The model under review builds one solid part; all positions refer to its coordinate system, in mm. Face numbers are marked on the shaded views. A direction names the side the tool comes from. Coordinates: 2 decimals unless noted, no trailing zeros. Loops run counter-clockwise (first coordinate to the right, second up) from the corner with the lowest first, then second, coordinate; pieces in that order, holes last. Notation, with made-up numbers: (14.25, 24.5) - (49.25, 24.5) arc R14 ccw to (49.25, 30.5) - close; hole circle Ø6 at (54, -11). An arc over 180 degrees is marked (long way). Answer in a Markdown table with one row per item. Add a question column.
(1) For line 1 along X through (y, z) = (55, 6); line 2 along X through (y, z) = (40, 4.25); line 3 along Y through (x, z) = (21, 1.35), list the stretches that pass through material, from the lowest coordinate up.
(2) We need section D-D on x = 21. Write out the cut boundary in (y, z).
(3) We need section A-A on z = 1.5. Give the number of separate pieces and of enclosed holes in the cut face, plus the area to 3 significant figures.
(4) We need section C-C on y = 30. Write out the cut boundary in (x, z).
(5) We need section B-B on x = 41. Write out the cut boundary in (y, z).
(6) Machinability: for the marked faces 4, 5 and 6, which of the approach directions +Z, -Z, +X, -X, +Y, -Y give a long, thin tool a straight path to every point of the face, cutting with its end or side? Answer none if there is none.
(7) For P1, Ø1.9, axis at x = 70, y = 20.5, coming from the -Z side; P2, Ø5.5, axis at x = 21, y = 69, coming from the +Z side; P3, Ø1.5, axis at x = 9, z = 4, coming from the +Y side; P4, Ø2.5, axis at x = 21, y = 9, coming from the -Z side, all flat-tipped, find the tip position at first contact; note any pin that passes through.
(8) Mouldability with a two-part tool opening along X and no side actions: class the marked faces 1, 2 and 3 as +X half, -X half, draft (parallel to the pull), parting line (faces both ways), or undercut.
from build123d import *

# Parameters (mm, degrees)
F1_DEPTH  = 8.5
F2_W      = 70
F2_H      = 68
F2_R      = 30
F3_DEPTH  = 4
F5_DEPTH  = 25
F6_R      = 3.2
F6_R_2    = 1.7
F7_DEPTH  = 3.1
F8_R      = 1.65
F9_DEPTH  = 25
F10_R     = 3.15
F11_DEPTH = 3.1
F13_DEPTH = 25


with BuildPart() as f1:
    # F0 (on Top) → F1 (new body)
    with BuildSketch(Plane.XY):
        with BuildLine():
            Line((0, 78), (0, 39))
            Line((0, 39), (11, 39))
            ThreePointArc((11, 39), (41, 69), (71, 39))
            Line((71, 39), (82, 39))
            Line((82, 39), (82, 78))
            Line((82, 78), (81, 78))
            ThreePointArc((81, 78), (79.535534, 74.464466), (76, 73))
            Line((76, 73), (6, 73))
            ThreePointArc((6, 73), (2.464466, 74.464466), (1, 78))
            Line((1, 78), (0, 78))
        make_face()
        with BuildLine():
            Line((0, 39), (0, 0))
            Line((0, 0), (1, 0))
            ThreePointArc((1, 0), (2.464466, 3.535534), (6, 5))
            Line((6, 5), (76, 5))
            ThreePointArc((76, 5), (79.535534, 3.535534), (81, 0))
            Line((81, 0), (82, 0))
            Line((82, 0), (82, 39))
            Line((82, 39), (71, 39))
            ThreePointArc((71, 39), (41, 9), (11, 39))
            Line((11, 39), (0, 39))
        make_face()
    extrude(amount=F1_DEPTH)

    # F2 (on face) → F3 (cut)
    with BuildSketch(Plane.XY.offset(8.5)):
        with Locations((41, 39)):
            Rectangle(F2_W, F2_H)
        with Locations((41, 39)):
            Circle(F2_R, mode=Mode.SUBTRACT)
    extrude(amount=-F3_DEPTH, mode=Mode.SUBTRACT)

    # F4 (on face) → F5 (cut)
    with BuildSketch(Plane(origin=(0, 0, 0), x_dir=(1, 0, 0), z_dir=(0, 0, -1))):
        with BuildLine():
            ThreePointArc((14.2, -19), (11.297918, -17.797918), (12.5, -20.7))
            ThreePointArc((12.5, -20.7), (13.702082, -20.202082), (14.2, -19))
        make_face()
        with BuildLine():
            ThreePointArc((14.2, -59), (13.702082, -57.797918), (12.5, -57.3))
            ThreePointArc((12.5, -57.3), (11.297918, -60.202082), (14.2, -59))
        make_face()
        with BuildLine():
            ThreePointArc((71.2, -59), (70.702082, -57.797918), (69.5, -57.3))
            ThreePointArc((69.5, -57.3), (68.297918, -60.202082), (71.2, -59))
        make_face()
        with BuildLine():
            ThreePointArc((71.2, -19), (69.5, -17.3), (67.8, -19))
            ThreePointArc((67.8, -19), (68.297918, -20.202082), (69.5, -20.7))
            ThreePointArc((69.5, -20.7), (70.702082, -20.202082), (71.2, -19))
        make_face()
    extrude(amount=-F5_DEPTH, mode=Mode.SUBTRACT)

    # F6 (on face) → F7 (cut)
    with BuildSketch(Plane(origin=(0, 0, 0), x_dir=(1, 0, 0), z_dir=(0, 0, -1))):
        with Locations((12.5, -19)):
            Circle(F6_R)
        with Locations((12.5, -19)):
            Circle(F6_R_2, mode=Mode.SUBTRACT)
        with Locations((12.5, -59)):
            Circle(F6_R)
        with Locations((12.5, -59)):
            Circle(F6_R_2, mode=Mode.SUBTRACT)
        with Locations((69.5, -19)):
            Circle(F6_R)
        with Locations((69.5, -19)):
            Circle(F6_R_2, mode=Mode.SUBTRACT)
        with Locations((69.5, -59)):
            Circle(F6_R)
        with Locations((69.5, -59)):
            Circle(F6_R_2, mode=Mode.SUBTRACT)
    extrude(amount=-F7_DEPTH, mode=Mode.SUBTRACT)

    # F8 (on face) → F9 (cut)
    with BuildSketch(Plane(origin=(0, 0, 0), x_dir=(1, 0, 0), z_dir=(0, 0, -1))):
        with Locations((21, -69)):
            Circle(F8_R)
        with BuildLine():
            ThreePointArc((62.65, -69), (62.166726, -67.833274), (61, -67.35))
            Line((61, -67.35), (61, -69))
            Line((61, -69), (59.35, -69))
            ThreePointArc((59.35, -69), (61, -70.65), (62.65, -69))
        make_face()
        with BuildLine():
            Line((61, -69), (61, -67.35))
            ThreePointArc((61, -67.35), (59.833274, -67.833274), (59.35, -69))
            Line((59.35, -69), (61, -69))
        make_face()
        with BuildLine():
            ThreePointArc((62.65, -9), (61, -7.35), (59.35, -9))
            Line((59.35, -9), (61, -9))
            Line((61, -9), (61, -10.65))
            ThreePointArc((61, -10.65), (62.166726, -10.166726), (62.65, -9))
        make_face()
        with BuildLine():
            Line((61, -9), (59.35, -9))
            ThreePointArc((59.35, -9), (59.833274, -10.166726), (61, -10.65))
            Line((61, -10.65), (61, -9))
        make_face()
        with Locations((21, -9)):
            Circle(F8_R)
    extrude(amount=-F9_DEPTH, mode=Mode.SUBTRACT)

    # F10 (on face) → F11 (cut)
    with BuildSketch(Plane(origin=(0, 0, 0), x_dir=(1, 0, 0), z_dir=(0, 0, -1))):
        with Locations((21, -9)):
            Circle(F10_R)
        with Locations((61, -9)):
            Circle(F10_R)
        with Locations((61, -69)):
            Circle(F10_R)
        with Locations((21, -69)):
            Circle(F10_R)
    extrude(amount=-F11_DEPTH, mode=Mode.SUBTRACT)

    # F12 (on face) → F13 (cut)
    with BuildSketch(Plane(origin=(0, 0, 0), x_dir=(1, 0, 0), z_dir=(0, 0, -1))):
        with BuildLine():
            ThreePointArc((12.5, -9), (9.93934, -7.93934), (11, -10.5))
            Line((11, -10.5), (11, -9))
            Line((11, -9), (12.5, -9))
        make_face()
        with BuildLine():
            Line((11, -9), (11, -10.5))
            ThreePointArc((11, -10.5), (12.06066, -10.06066), (12.5, -9))
            Line((12.5, -9), (11, -9))
        make_face()
        with BuildLine():
            ThreePointArc((69.5, -9), (69.93934, -10.06066), (71, -10.5))
            Line((71, -10.5), (71, -9))
            Line((71, -9), (69.5, -9))
        make_face()
        with BuildLine():
            Line((71, -9), (71, -10.5))
            ThreePointArc((71, -10.5), (72.06066, -10.06066), (72.5, -9))
            ThreePointArc((72.5, -9), (71, -7.5), (69.5, -9))
            Line((69.5, -9), (71, -9))
        make_face()
        with BuildLine():
            ThreePointArc((71, -67.5), (69.93934, -67.93934), (69.5, -69))
            Line((69.5, -69), (71, -69))
            Line((71, -69), (71, -67.5))
        make_face()
        with BuildLine():
            Line((71, -69), (69.5, -69))
            ThreePointArc((69.5, -69), (71, -70.5), (72.5, -69))
            ThreePointArc((72.5, -69), (72.06066, -67.93934), (71, -67.5))
            Line((71, -67.5), (71, -69))
        make_face()
        with BuildLine():
            ThreePointArc((11, -67.5), (9.93934, -70.06066), (12.5, -69))
            Line((12.5, -69), (11, -69))
            Line((11, -69), (11, -67.5))
        make_face()
        with BuildLine():
            Line((11, -69), (12.5, -69))
            ThreePointArc((12.5, -69), (12.06066, -67.93934), (11, -67.5))
            Line((11, -67.5), (11, -69))
        make_face()
    extrude(amount=-F13_DEPTH, mode=Mode.SUBTRACT)


solid = f1.part
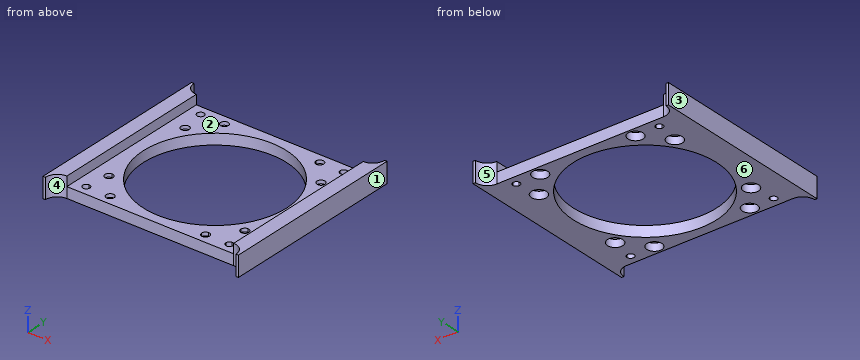
Outcome:
| question | item | result |
|---|---|---|
| 1 | line 1 | 0 to 6, 76 to 82 |
| 1 | line 2 | 0 to 11.02, 70.98 to 82 |
| 1 | line 3 | 5 to 5.85, 12.15 to 16.64, 61.36 to 65.85, 72.15 to 73 |
| 2 | outline | (5, 0) - (5.85, 0) - (5.85, 3.1) - (7.35, 3.1) - (7.35, 4.5) - (5, 4.5) - close; (10.65, 3.1) - (12.15, 3.1) - (12.15, 0) - (16.64, 0) - (16.64, 4.5) - (10.65, 4.5) - close; (61.36, 0) - (65.85, 0) - (65.85, 3.1) - (67.35, 3.1) - (67.35, 4.5) - (61.36, 4.5) - close; (70.65, 3.1) - (72.15, 3.1) - (72.15, 0) - (73, 0) - (73, 4.5) - (70.65, 4.5) - close |
| 3 | separate pieces | 1 |
| 3 | enclosed holes | 13 |
| 3 | area | 2,510 mm² |
| 4 | outline | (0, 0) - (12.38, 0) - (12.38, 4.5) - (6, 4.5) - (6, 8.5) - (0, 8.5) - close; (69.62, 0) - (82, 0) - (82, 8.5) - (76, 8.5) - (76, 4.5) - (69.62, 4.5) - close |
| 5 | outline | (5, 0) - (9, 0) - (9, 4.5) - (5, 4.5) - close; (69, 0) - (73, 0) - (73, 4.5) - (69, 4.5) - close |
| 6 | face 4 | +Z, -Z, -Y |
| 6 | face 5 | +Z, -Z, +Y |
| 6 | face 6 | -Z, +X, -X, +Y, -Y |
| 7 | P1 | z = 3.1 |
| 7 | P2 | z = 4.5 |
| 7 | P3 | y = 73 |
| 7 | P4 | through |
| 8 | face 1 | +X half |
| 8 | face 2 | undercut |
| 8 | face 3 | -X half |
